Build history of the part. All positions in model axes, mm. Round coordinates to 2 decimals unless told otherwise and drop trailing zeros. Loops run counter-clockwise (first coordinate to the right, second up) from the corner with the lowest first, then second, coordinate; pieces in that order, holes last. Notation, with made-up numbers: (85.25, 11.5) -> (123.25, 11.5) arc R14 cw to (123.25, 24.5) -> close; hole circle Ø2 at (-11, 21.25). An arc over 180 degrees is marked (long way). Put each result on its own line as item: value. Start each with the question number.
Item 1: Cut at C-C, the plane y = -4.5. List the corners of the cut face in (x, z), plus the area to 3 significant figures.
Item 2: Drill centre lines: probe 1 along X at (y, z) = (5.5, 60.5); probe 2 along Z at (x, y) = (1.75, 5.5); probe 3 along X at (y, z) = (3.75, 9.5). Where is each one in solid material? Low to high. Write a range as [from, to].
Item 3: Cut at D-D, the plane z = 11.5. List the corners of the cut face in (x, y), plus the area to 3 significant figures.
Item 4: Cut at A-A, the plane z = 58. List the corners of the cut face in (x, y), plus the area to 3 significant figures.
Item 5: Cut at B-B, the plane x = 0. List the corners of the cut face in (y, z), plus the area to 4 significant figures.
Item 6: Flat gauge pins, fed straight in: pin 1 Ø2 at (y, z) = (5, 60) entering from -X; pin 2 Ø2.5 at (x, z) = (0.5, 62) entering from +Y; pin 3 Ø0.6 at (y, z) = (5.5, 54) entering from +X. Where does each tip first touch, or does it go through?
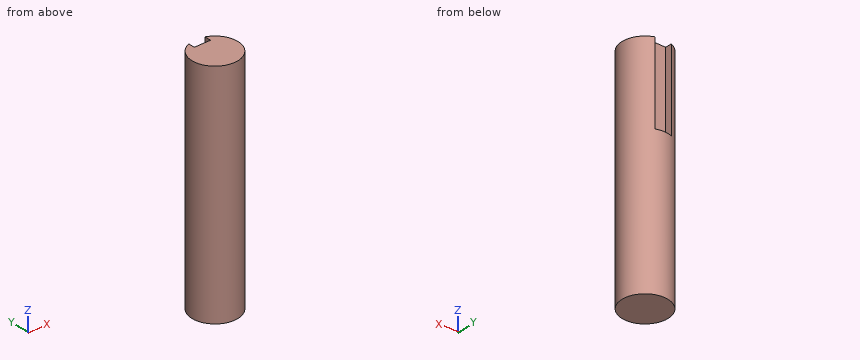
```python
from build123d import *

# Parameters (mm, degrees)
SKETCH1_R           = 7
BOSS_EXTRUDE1_DEPTH = 70
CUT_EXTRUDE1_START  = -25
CUT_EXTRUDE1_DEPTH  = 25


with BuildPart() as part:
    # Sketch1 → Boss-Extrude1 (new body)
    with BuildSketch(Plane.XY):
        Circle(SKETCH1_R)
    extrude(amount=BOSS_EXTRUDE1_DEPTH)

    # Sketch2 → Cut-Extrude1 (cut)
    with BuildSketch(Plane.XY.offset(70).offset(CUT_EXTRUDE1_START)):
        with BuildLine():
            Line((-2.5, 4.5), (2.5, 4.5))
            Line((2.5, 4.5), (2.5, 6.538348415))
            ThreePointArc((2.5, 6.538348415), (0, 7), (-2.5, 6.538348415))
            Line((-2.5, 6.538348415), (-2.5, 4.5))
        make_face()
    extrude(amount=CUT_EXTRUDE1_DEPTH, mode=Mode.SUBTRACT)


solid = part.part
```
Reply:
1. outline: (-5.36, 0) -> (5.36, 0) -> (5.36, 70) -> (-5.36, 70) -> close
1. area: 751 mm^2
2. probe 1: x = [-4.33, -2.5], [2.5, 4.33]
2. probe 2: z = [0, 45]
2. probe 3: x = [-5.91, 5.91]
3. outline: circle Ø14 at (0, 0)
3. area: 154 mm^2
4. outline: (-2.5, 4.5) -> (-2.5, 6.54) arc R7 ccw (long way) to (2.5, 6.54) -> (2.5, 4.5) -> close
4. area: 142 mm^2
5. outline: (-7, 0) -> (7, 0) -> (7, 45) -> (4.5, 45) -> (4.5, 70) -> (-7, 70) -> close
5. area: 917.5 mm^2
6. pin 1: stops at x = -5.74
6. pin 2: stops at y = 4.5
6. pin 3: stops at x = 4.69
